```python
from build123d import *

# Parameters (mm, degrees)
SKETCH1_W                 = 32.5
SKETCH1_H                 = 48
BOSS_EXTRUDE1_DEPTH       = 3
F_2_56_TAPPED_HOLE1_D     = 1.778
F_2_56_TAPPED_HOLE1_DEPTH = 7.46583491
F_2_56_TAPPED_HOLE1_TIP   = 0.53416509
F_2_56_TAPPED_HOLE2_D     = 1.778
F_2_56_TAPPED_HOLE2_DEPTH = 7.46583491
F_2_56_TAPPED_HOLE2_TIP   = 0.53416509
CUT_EXTRUDE2_DEPTH        = 1.5
SKETCH10_R                = 3.5
CUT_EXTRUDE3_DEPTH        = 3


with BuildPart() as part:
    # Sketch1 → Boss-Extrude1 (new body)
    with BuildSketch(Plane(origin=(0, 0, 0), x_dir=(1, 0, 0), z_dir=(0, 1, 0))):
        with Locations((16.25, 24)):
            Rectangle(SKETCH1_W, SKETCH1_H)
    extrude(amount=BOSS_EXTRUDE1_DEPTH)

    # #2-56 Tapped Hole1
    with Locations(Plane.ZY):
        with Locations((-36, 1.5), (-12, 1.5)):
            Hole(F_2_56_TAPPED_HOLE1_D / 2, depth=F_2_56_TAPPED_HOLE1_DEPTH)
            with Locations((0, 0, -(F_2_56_TAPPED_HOLE1_DEPTH + F_2_56_TAPPED_HOLE1_TIP / 2))):  # 118° drill point
                Cone(0, F_2_56_TAPPED_HOLE1_D / 2, F_2_56_TAPPED_HOLE1_TIP, mode=Mode.SUBTRACT)

    # #2-56 Tapped Hole2
    with Locations(Plane(origin=(32.5, 0, 0), x_dir=(0, 0, -1), z_dir=(1, 0, 0))):
        with Locations((12, 1.5), (36, 1.5)):
            Hole(F_2_56_TAPPED_HOLE2_D / 2, depth=F_2_56_TAPPED_HOLE2_DEPTH)
            with Locations((0, 0, -(F_2_56_TAPPED_HOLE2_DEPTH + F_2_56_TAPPED_HOLE2_TIP / 2))):  # 118° drill point
                Cone(0, F_2_56_TAPPED_HOLE2_D / 2, F_2_56_TAPPED_HOLE2_TIP, mode=Mode.SUBTRACT)

    # Sketch11 → Cut-Extrude2 (cut)
    with BuildSketch(Plane(origin=(0, 0, 0), x_dir=(-1, 0, 0), z_dir=(0, -1, 0))):
        Polygon((-21.05, 4.57), (-21.05, 8.57), (-11.45, 8.57), (-11.45, 0.57), (-21.05, 0.57), align=None)
    extrude(amount=-CUT_EXTRUDE2_DEPTH, mode=Mode.SUBTRACT)

    # Sketch10 → Cut-Extrude3 (cut)
    with BuildSketch(Plane(origin=(0, 3, 0), x_dir=(1, 0, 0), z_dir=(0, 1, 0))):
        with Locations(Location((16.25, 4.57, 0), (0, 0, 270))):
            Circle(SKETCH10_R)
    extrude(amount=-CUT_EXTRUDE3_DEPTH, mode=Mode.SUBTRACT)


solid = part.part
```
CAD build for the part. Positions are in the model's coordinates, mm. A direction names the side the tool comes from. Round coordinates to 2 decimals unless told otherwise and drop trailing zeros. Order: outer loops, then holes, each group sorted by start corner. A loop starts at its lowest first (then second) coordinate and runs counter-clockwise, first axis right, second up. Notation, with made-up numbers: (-22, 39.25) - (25, 39.25) arc R27 ccw to (25, 65.25) - close; hole circle Ø10 at (-29, 61.25). An arc over 180 degrees is marked (long way). Answer in a Markdown table with one row per item. Add a question column.
(1) Probe L1, parallel to Z at x = 29, y = 1.5; L2, parallel to X at y = 1.05, z = -4.5; L3, parallel to Y at x = 1.75, z = -36. List the from-to ranges inside material, lowest first. Write a range as [from, to].
(2) 3-axis set-ups, long thin cutter, end or side, ignore diameter. For faces 1 (the face through (19.72, 2.26, -5.03)), 2 (the face through (3.79, 1.54, -35.11)), 3 (the face through (11.45, 1, -5)), 4 (the face through (28.715, 2.101, -12.655)): which of +Z, -Z, +X, -X, +Y, -Y reach the whole face in a straight line?
(3) Drop a flat-ended pin along its axis: pin 1 Ø1.1 at (y, z) = (1.5, -36) entering from +X. Give the stop position or say it passes through.
(4) Band-saw the part on C-C on x = 5. List the corners of the cut face in (y, z).
(5) Band-saw the part on B-B on x = 14. List the corners of the cut face in (y, z), and give its area (3 significant figures).
(6) Mould opens along Y. For faces 5 (the face through (7.91, 1.44, -11.86)), 6 (the face through (28.71, 1.54, -36.89)), 7 (the face through (21.05, 1, -5)), 8 (the face through (16, 3, -24)) say: +Y half, -Y half, draft (parallel to the pull), parting line (faces both ways), or undercut.
(7) Band-saw the part on A-A on z = -4.57. List the corners of the cut face in (x, y), and give its area (3 significant figures).
Data:
| question | item | result |
|---|---|---|
| 1 | L1 | z = [-48, -36.89], [-35.11, -12.89], [-11.11, 0] |
| 1 | L2 | x = [0, 11.45], [21.05, 32.5] |
| 1 | L3 | y = [0, 0.61], [2.39, 3] |
| 2 | face 1 | +Y, -Y |
| 2 | face 2 | -X |
| 2 | face 3 | -Y |
| 2 | face 4 | +X |
| 3 | pin 1 | stops at x = 24.83 |
| 4 | outline | (0, -48) - (3, -48) - (3, 0) - (0, 0) - close; hole circle Ø1.78 at (1.5, -36); hole circle Ø1.78 at (1.5, -12) |
| 5 | outline | (0, -48) - (3, -48) - (3, -7.25) - (1.5, -7.25) - (1.5, -8.57) - (0, -8.57) - close; (0, -0.57) - (1.5, -0.57) - (1.5, -1.89) - (3, -1.89) - (3, 0) - (0, 0) - close |
| 5 | area | 124 mm^2 |
| 6 | face 5 | undercut |
| 6 | face 6 | undercut |
| 6 | face 7 | draft |
| 6 | face 8 | +Y half |
| 7 | outline | (0, 0) - (11.45, 0) - (11.45, 1.5) - (12.75, 1.5) - (12.75, 3) - (0, 3) - close; (19.75, 1.5) - (21.05, 1.5) - (21.05, 0) - (32.5, 0) - (32.5, 3) - (19.75, 3) - close |
| 7 | area | 72.6 mm^2 |
